```python
from build123d import *

# Parameters (mm, degrees)
BOSS_EXTRU_1_DEPTH                  = 22
BOSS_EXTRU_1_DEPTH_BACK             = 22
BOSS_EXTRU_5_START                  = 22
BOSS_EXTRU_5_DEPTH                  = 1
BOSS_EXTRU_6_START                  = -22
BOSS_EXTRU_6_DEPTH                  = 1
BOSS_EXTRU_7_DEPTH                  = 2
BOSS_EXTRU_8_DEPTH                  = 2
CONG_1_R                            = 1
ENL_V_MAT_EXTRU_1_REACH             = 39.042
ESQUISSE6_R                         = 0.75
ESQUISSE6_W                         = 23.5
ESQUISSE6_H                         = 23.5
ENL_V_MAT_EXTRU_1_DIRECTION_2_DEPTH = 2


with BuildPart() as part:
    # Esquisse1 → Boss.-Extru.1 (new body, two sides)
    with BuildSketch(Plane.XY) as boss_extru_1_sk:
        Polygon((0, 38.384776311), (28.384776311, 38.384776311), (28.384776311, 18.384776311), (10, 0), (0, 0), (0, 1), (9.585786438, 1), (27.384776311, 18.798989873), (27.384776311, 37.384776311), (0, 37.384776311), align=None)
    extrude(amount=BOSS_EXTRU_1_DEPTH)
    extrude(boss_extru_1_sk.sketch, amount=-BOSS_EXTRU_1_DEPTH_BACK)

    # Esquisse2 → Boss.-Extru.5 (add)
    with BuildSketch(Plane.XY.offset(BOSS_EXTRU_5_START)):
        Polygon((28.384776311, 18.384776311), (28.384776311, 38.384776311), (0, 38.384776311), (0, 0), (10, 0), align=None)
    extrude(amount=BOSS_EXTRU_5_DEPTH)

    # Esquisse3 → Boss.-Extru.6 (add)
    with BuildSketch(Plane.XY.offset(BOSS_EXTRU_6_START)):
        Polygon((0, 38.384776311), (0, 0), (10, 0), (28.384776311, 18.384776311), (28.384776311, 38.384776311), align=None)
    extrude(amount=-BOSS_EXTRU_6_DEPTH)

    # Esquisse4 → Boss.-Extru.7 (add)
    with BuildSketch(Plane(origin=(0, 38.384776311, 0), x_dir=(1, 0, 0), z_dir=(0, 1, 0))):
        Polygon((11.01040764, 19.445436483), (13.838834765, 16.617009358), (16.66726189, 19.445436483), (13.838834765, 22.273863607), align=None)
        Polygon((15.960155108, -20.859650045), (18.788582233, -18.03122292), (15.960155108, -15.202795796), (13.131727984, -18.03122292), align=None)
    extrude(amount=BOSS_EXTRU_7_DEPTH)

    # Esquisse5 → Boss.-Extru.8 (add)
    with BuildSketch(Plane(origin=(0, 40.384776311, 0), x_dir=(1, 0, 0), z_dir=(0, 1, 0))):
        Polygon((13.838834765, 22.273863607), (16.66726189, 19.445436483), (8.889087297, 11.66726189), (6.060660172, 14.495689014), align=None)
        Polygon((13.131727984, -18.03122292), (15.960155108, -20.859650045), (23.738329701, -13.081475452), (20.909902577, -10.253048327), align=None)
    extrude(amount=BOSS_EXTRU_8_DEPTH)

    # Cong_1
    cong_1_edges = [part.edges().sort_by_distance(p)[0] for p in [
        (20.909902577, 41.384776311, 10.253048327),
        (23.738329701, 41.384776311, 13.081475452),
        (6.060660172, 41.384776311, -14.495689014),
        (8.889087297, 41.384776311, -11.66726189),
        (13.838834765, 40.384776311, -22.273863607),
        (16.66726189, 40.384776311, -19.445436483),
        (13.131727984, 40.384776311, 18.03122292),
        (15.960155108, 40.384776311, 20.859650045),
    ]]
    fillet(cong_1_edges, radius=CONG_1_R)

    # Esquisse6 → Enl_v. mat.-Extru.1 (cut, up to next)
    with BuildSketch(Plane(origin=(5, -5, 0), x_dir=(0, 0, -1), z_dir=(0.707106781, -0.707106781, 0)), mode=Mode.PRIVATE) as enl_v_mat_extru_1_sk1:
        with Locations((14.25, 20.071067812)):
            Circle(ESQUISSE6_R)
    enl_v_mat_extru_1_tool1 = extrude(enl_v_mat_extru_1_sk1.sketch, amount=-ENL_V_MAT_EXTRU_1_REACH, mode=Mode.PRIVATE) & part.part
    add(enl_v_mat_extru_1_tool1.solids().sort_by_distance((19.192388, 9.192388, -14.25))[0], mode=Mode.SUBTRACT)
    # Esquisse6 → Enl_v. mat.-Extru.1 (cut, up to next)
    with BuildSketch(Plane(origin=(5, -5, 0), x_dir=(0, 0, -1), z_dir=(0.707106781, -0.707106781, 0)), mode=Mode.PRIVATE) as enl_v_mat_extru_1_sk2:
        with Locations((-14.25, 20.071067812)):
            Circle(ESQUISSE6_R)
    enl_v_mat_extru_1_tool2 = extrude(enl_v_mat_extru_1_sk2.sketch, amount=-ENL_V_MAT_EXTRU_1_REACH, mode=Mode.PRIVATE) & part.part
    add(enl_v_mat_extru_1_tool2.solids().sort_by_distance((19.192388, 9.192388, 14.25))[0], mode=Mode.SUBTRACT)
    # Esquisse6 → Enl_v. mat.-Extru.1 (cut, up to next)
    with BuildSketch(Plane(origin=(5, -5, 0), x_dir=(0, 0, -1), z_dir=(0.707106781, -0.707106781, 0)), mode=Mode.PRIVATE) as enl_v_mat_extru_1_sk3:
        with Locations((0, 20.071067812)):
            Rectangle(ESQUISSE6_W, ESQUISSE6_H)
    enl_v_mat_extru_1_tool3 = extrude(enl_v_mat_extru_1_sk3.sketch, amount=-ENL_V_MAT_EXTRU_1_REACH, mode=Mode.PRIVATE) & part.part
    add(enl_v_mat_extru_1_tool3.solids().sort_by_distance((19.192388, 9.192388, 0))[0], mode=Mode.SUBTRACT)

    # Esquisse6 → Enl_v. mat.-Extru.1 direction 2 (cut)
    with BuildSketch(Plane(origin=(5, -5, 0), x_dir=(0, 0, -1), z_dir=(0.707106781, -0.707106781, 0))):
        with Locations((14.25, 20.071067812)):
            Circle(ESQUISSE6_R)
        with Locations((-14.25, 20.071067812)):
            Circle(ESQUISSE6_R)
        with Locations((0, 20.071067812)):
            Rectangle(ESQUISSE6_W, ESQUISSE6_H)
    extrude(amount=ENL_V_MAT_EXTRU_1_DIRECTION_2_DEPTH, mode=Mode.SUBTRACT)


solid = part.part
```
Geometry check sheet. Reference: the model listing, model coordinates, mm. A direction names the side the tool comes from. Give positions to 0.01 mm unless a question says otherwise; leave off trailing zeros. Order: outer loops, then holes, each group sorted by start corner. A loop starts at its lowest first (then second) coordinate and runs counter-clockwise, first axis right, second up.
1. Section check D-D, the plane y = 25. Enter the section's corners in (x, z).
2. Release check for a two-part mould opening along Y. For faces 1 (the face through (19, 9, 16)), 2 (the face through (5, 1, 0)), 3 (the face through (19.1, 40.8, 17.72)) record: pulls with the +Y half, pulls with the -Y half, needs draft (parallel to the pull), parting line crosses it, or undercut.
3. Section check B-B, the plane x = 4.5. Enter the section's corners in (y, z), and give its area (3 significant figures).
4. Access from +Z, -Z, +X, -X, +Y, -Y to the whole of each face (thin tool, end or side, straight path). Record for faces 4 (the face through (22.334, 41.371, 11.677)), 5 (the face through (13.53, 40.8, -16.31)), 6 (the face through (13.85, 40.41, -21.86)), 7 (the face through (15.949, 40.357, 20.445)), 8 (the face through (14, 23, 22)).
5. Thickness scan on L1, parallel to Z at x = 16, y = 20; L2, parallel to Y at x = 3.5, z = 1; L3, parallel to Y at x = 11, z = -16.5. Record the ranges inside material, lowest first.
6. Gauge pin test, flat ends, axial feed: pin 1 Ø8 at (x, z) = (20.5, 15.5) entering from -Y; pin 2 Ø2 at (x, z) = (17, 14.5) entering from -Y; pin 3 Ø10 at (x, z) = (21, 4.5) entering from -Y. Record the tip position at first contact, or that the pin passes through.
7. Section check C-C, the plane y = 14. Enter the section's corners in (x, z), and give its area (3 significant figures).
8. Section check A-A, the plane z = 7. Enter the section's corners in (x, y), and give its area (3 significant figures).
Values follow:
1. outline: (0, -23) - (28.38, -23) - (28.38, 23) - (0, 23) - (0, 22) - (27.38, 22) - (27.38, -22) - (0, -22) - close
2. face 1: pulls with the -Y half
2. face 2: undercut
2. face 3: needs draft
3. outline: (0, -23) - (38.38, -23) - (38.38, 23) - (0, 23) - close; hole (1, -22) - (37.38, -22) - (37.38, 22) - (1, 22) - close
3. area: 165 mm2
4. face 4: -Z, +X, +Y
4. face 5: +X, +Y
4. face 6: -Z, +Y
4. face 7: +Z, +Y
4. face 8: -X
5. L1: z = -23 to -22, 22 to 23
5. L2: y = 0 to 1, 37.38 to 38.38
5. L3: y = 1 to 2.41, 37.38 to 38.38, 40.38 to 42.38
6. pin 1: stops at y = 6.5
6. pin 2: stops at y = 6
6. pin 3: stops at y = 37.38
7. outline: (0, -23) - (24, -23) - (24, -11.75) - (22.59, -11.75) - (22.59, -22) - (0, -22) - close; (0, 22) - (22.59, 22) - (22.59, 11.75) - (24, 11.75) - (24, 23) - (0, 23) - close
7. area: 77.0 mm2
8. outline: (0, 0) - (10, 0) - (10.88, 0.88) - (10.18, 1.59) - (9.59, 1) - (0, 1) - close; (0, 37.38) - (27.38, 37.38) - (27.38, 18.8) - (26.79, 18.21) - (27.5, 17.5) - (28.38, 18.38) - (28.38, 38.38) - (0, 38.38) - close
8. area: 59.1 mm2
